```python
from build123d import *

# Parameters (mm, degrees)
F1_DEPTH      = 1872.45625
F3_DEPTH      = 38.101
F3_DEPTH_BACK = 38.101


with BuildPart() as f1:
    # F0 (on Top) → F1 (new body)
    with BuildSketch(Plane.XY):
        with BuildLine():
            ThreePointArc((-38.1, -28.575), (-35.3101920908, -35.3101920908), (-28.575, -38.1))
            Line((-28.575, -38.1), (28.575, -38.1))
            ThreePointArc((28.575, -38.1), (35.3101920908, -35.3101920908), (38.1, -28.575))
            Line((38.1, -28.575), (38.1, 28.575))
            ThreePointArc((38.1, 28.575), (35.3101920908, 35.3101920908), (28.575, 38.1))
            Line((28.575, 38.1), (-28.575, 38.1))
            ThreePointArc((-28.575, 38.1), (-35.3101920908, 35.3101920908), (-38.1, 28.575))
            Line((-38.1, 28.575), (-38.1, -28.575))
        make_face()
        with BuildLine():
            Line((28.575, -33.3375), (-28.575, -33.3375))
            ThreePointArc((-28.575, -33.3375), (-31.9425960454, -31.9425960454), (-33.3375, -28.575))
            Line((-33.3375, -28.575), (-33.3375, 28.575))
            ThreePointArc((-33.3375, 28.575), (-31.9425960454, 31.9425960454), (-28.575, 33.3375))
            Line((-28.575, 33.3375), (28.575, 33.3375))
            ThreePointArc((28.575, 33.3375), (31.9425960454, 31.9425960454), (33.3375, 28.575))
            Line((33.3375, 28.575), (33.3375, -28.575))
            ThreePointArc((33.3375, -28.575), (31.9425960454, -31.9425960454), (28.575, -33.3375))
        make_face(mode=Mode.SUBTRACT)
    extrude(amount=F1_DEPTH)

    # F2 (on Right) → F3 (cut, two sides)
    with BuildSketch(Plane.YZ) as f3_sk:
        Polygon((-38.1, 76.2), (-38.1, 0), (38.1, 0), align=None)
        Polygon((38.1, 1872.45625), (-38.1, 1872.45625), (38.1, 1796.25625), align=None)
    extrude(amount=-F3_DEPTH, mode=Mode.SUBTRACT)
    extrude(f3_sk.sketch, amount=F3_DEPTH_BACK, mode=Mode.SUBTRACT)


solid = f1.part
```
The listing builds one solid part. Answer for the finished solid, in the listing's coordinates (mm). A direction names the side the tool comes from. Give positions to 0.01 mm unless a question says otherwise; leave off trailing zeros. Write each loop counter-clockwise with the first axis right and the second up, starting at its lowest first coordinate (ties: lowest second). Pieces come first, ordered by that corner, then holes. Notation, with made-up numbers: M 63,-38.5 L 93,-38.5 A29 ccw 93,0.5 Z; hole C 40.25,-29.75 d7. An arc over 180 degrees is marked long. Write each question's results on one line, items separated by ' | '.
Q1. Section B-B, the plane x = -17 is taken. Write down the section's boundary in (y, z), then the cut area to 3 significant figures.
Output values:
outline: M -38.1,76.2 L -33.34,71.44 L -33.34,1867.69 L -38.1,1872.46 Z; M 33.34,4.76 L 38.1,0 L 38.1,1796.26 L 33.34,1801.02 Z | area: 17,100 mm2
Q2. Section C-C, the plane y = -7 is taken. Write down the section's boundary in (x, z), then the cut area to 3 significant figures.
Output values:
outline: M -38.1,45.1 L -33.34,45.1 L -33.34,1841.36 L -38.1,1841.36 Z; M 33.34,45.1 L 38.1,45.1 L 38.1,1841.36 L 33.34,1841.36 Z | area: 17,100 mm2
Q3. Consider L1, parallel to X at y = 26, z = 1470.5; L2, parallel to Z at x = -33, y = -33. Determine where each line is inside the solid, lowest interval first. Write a range as from..to.
Output values:
L1: -38.1..-33.34, 33.34..38.1 | L2: 71.1..1867.36
Q4. For a pull along Y with two mould halves and no side action, classify faces 3 (the flat face through (-38.1, 0, 923)), 4 (the flat face through (0, -33.338, 957)), 5 (the flat face through (0, 38.1, 886)) as released by +Y, released by -Y, zero draft, split by the parting line, or undercut.
Output values:
face 3: zero draft | face 4: undercut | face 5: released by +Y
Q5. A tool of negligible diameter and unlimited length cuts with its end or side. For faces 1 (the flat face through (-33.7, 0.2, 37.9)), 2 (the flat face through (-33.338, 0, 923)), from which of +Z, -Z, +X, -X, +Y, -Y can it reach the whole face along a straight path? Write none if from no direction.
Output values:
face 1: -Z, +X, -X, -Y | face 2: +Z, -Z
